CAD build for the part. Positions are in the model's coordinates, mm. A direction names the side the tool comes from. Round coordinates to 2 decimals unless told otherwise and drop trailing zeros. Loops run counter-clockwise (first coordinate to the right, second up) from the corner with the lowest first, then second, coordinate; pieces in that order, holes last.
from build123d import *

# Parameters (mm, degrees)
EXTRUDE_1_DEPTH     = 10
SKETCH_2_W          = 10.780789019
SKETCH_2_H          = 10
CUT_EXTRUDE_1_DEPTH = 6
SKETCH_3_W          = 10
SKETCH_3_H          = 18.171763081
EXTRUDE_2_DEPTH     = 1
SKETCH_4_R          = 1.5
CUT_EXTRUDE_2_DEPTH = 11
SKETCH_5_W          = 11.719210981
SKETCH_5_H          = 10
CUT_EXTRUDE_3_DEPTH = 3.18


with BuildPart() as part:
    # 草图1 → 凸台-拉伸1 (new body)
    with BuildSketch(Plane.XY):
        Polygon((7.850374618, 8.603451253), (16.234951688, 8.603451253), (16.234951688, 16.628704923), (16.234951688, 20.775214334), (26.954162669, 20.775214334), (26.954162669, -17.403924352), (5.454162669, -17.403924352), (5.454162669, 8.603451253), align=None)
    extrude(amount=EXTRUDE_1_DEPTH)

    # 草图2 → 切除-拉伸1 (cut)
    with BuildSketch(Plane(origin=(0, 8.603451253, 0), x_dir=(1, 0, 0), z_dir=(0, 1, 0))):
        with Locations((10.844557179, -5)):
            Rectangle(SKETCH_2_W, SKETCH_2_H)
    extrude(amount=-CUT_EXTRUDE_1_DEPTH, mode=Mode.SUBTRACT)

    # 草图3 → 凸台-拉伸2 (add)
    with BuildSketch(Plane.ZY.offset(-16.234951688)):
        with Locations((5, 11.689332794)):
            Rectangle(SKETCH_3_W, SKETCH_3_H)
    extrude(amount=EXTRUDE_2_DEPTH)

    # 草图4 → 切除-拉伸2 (cut, through all)
    with BuildSketch(Plane.XY.offset(10)):
        with Locations((16.204162669, -9.403924352)):
            Circle(SKETCH_4_R)
        with Locations((22.454162669, 10.775214334)):
            Circle(SKETCH_4_R)
    extrude(amount=-CUT_EXTRUDE_2_DEPTH, mode=Mode.SUBTRACT)

    # 草图5 → 切除-拉伸3 (cut)
    with BuildSketch(Plane(origin=(0, 20.775214334, 0), x_dir=(1, 0, 0), z_dir=(0, 1, 0))):
        with Locations((21.094557179, -5)):
            Rectangle(SKETCH_5_W, SKETCH_5_H)
    extrude(amount=-CUT_EXTRUDE_3_DEPTH, mode=Mode.SUBTRACT)


solid = part.part
Item 1: Cut at D-D (y = 8). List the corners of the cut face in (x, z).
Verdict:
outline: (15.23, 0) - (26.95, 0) - (26.95, 10) - (15.23, 10) - close
Item 2: Wall check: L1, parallel to X at y = -9.5, z = 9.5; L2, parallel to Y at x = 11, z = 1.75; L3, parallel to X at y = 11.5, z = 3.25. Give the ranges that are in metal, low to high.
Verdict:
L1: x = 5.45 to 14.71, 17.7 to 26.95
L2: y = -17.4 to 2.6
L3: x = 15.23 to 21.14, 23.77 to 26.95
Item 3: Cut at B-B (z = 4.25). List the corners of the cut face in (x, y), plus the area to 3 significant figures.
Verdict:
outline: (5.45, -17.4) - (26.95, -17.4) - (26.95, 17.6) - (15.23, 17.6) - (15.23, 2.6) - (5.45, 2.6) - close; hole circle Ø3 at (16.2, -9.4); hole circle Ø3 at (22.45, 10.78)
area: 592 mm2
Item 4: 3-axis set-ups, long thin cutter, end or side, ignore diameter. For faces 5 (the flat face through (15.235, 10, 5)), 6 (the cylindrical face through (23.885, 11.226, 5.07)): which of +Z, -Z, +X, -X, +Y, -Y reach the whole face in a straight line?
Verdict:
face 5: +Z, -Z, -X, +Y
face 6: +Z, -Z
Item 5: Cut at C-C (x = 12.75). List the corners of the cut face in (y, z), plus the area to 3 significant figures.
Verdict:
outline: (-17.4, 0) - (2.6, 0) - (2.6, 10) - (-17.4, 10) - close
area: 200 mm2
Item 6: Cut at A-A (x = 22.5). List the corners of the cut face in (y, z).
Verdict:
outline: (-17.4, 0) - (9.28, 0) - (9.28, 10) - (-17.4, 10) - close; (12.27, 0) - (17.6, 0) - (17.6, 10) - (12.27, 10) - close
Item 7: Flat gauge pins, fed straight in: P1, Ø1, axis at y = 4, z = 3, coming from the -X side; P2, Ø4, axis at x = 12, y = 6.5, coming from the -Z side. Where does each tip first touch, or does it go through?
Verdict:
P1: stops at x = 15.23
P2: passes through
Item 8: Mould opens along Y. For faces 1 (the flat face through (10, 2.603, 5)), 2 (the flat face through (26.954, 0, 5)), 3 (the cylindrical face through (14.706, -9.338, 5.07)), 4 (the flat face through (16, -17.404, 5)) say: released by +Y, released by -Y, zero draft, split by the parting line, or undercut.
Verdict:
face 1: released by +Y
face 2: zero draft
face 3: undercut
face 4: released by -Y
